Can you work these out from the model? Positions are in its coordinate system, mm. Give positions to 0.01 mm unless a question says otherwise; leave off trailing zeros. Order: outer loops, then holes, each group sorted by start corner. A loop starts at its lowest first (then second) coordinate and runs counter-clockwise, first axis right, second up. Notation, with made-up numbers: M -1.5,-29.75 L 3.5,-29.75 A21 ccw 3.5,-19.75 Z; hole C 72,-34 d9. An arc over 180 degrees is marked long. One line per question, with ' | ' between items. Start each with the question number.
1) If we section it at A-A, the plane y = 6: Please give me the cut outline in (x, z), plus the area to 3 significant figures.
2) Please list where these lines run through material, in increasing order: line 1 along Z through (x, y) = (28, 2.75); line 2 along X through (y, z) = (7, -58); line 3 along Y through (x, z) = (18.5, -72). Write a range as [from, to].
3) I'm going to push flat-ended pins straight in: pin 1 Ø12 at (x, z) = (62.5, -54.5) entering from -Y; pin 2 Ø2 at (y, z) = (1, -73.5) entering from +X; pin 3 Ø4 at (x, y) = (25, 3.5) entering from +Z; pin 4 Ø5 at (y, z) = (8, -38) entering from -X. Where does each tip first touch, or does it pass through?
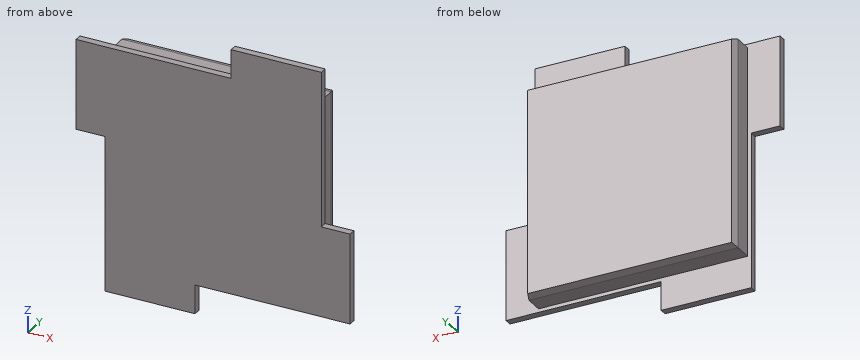
```python
from build123d import *

# Parameters (mm, degrees)
ESQUISSE1_W        = 8
ESQUISSE1_H        = 25
ESQUISSE1_W_2      = 25
ESQUISSE1_H_2      = 8
ESQUISSE1_W_3      = 60
ESQUISSE1_H_3      = 60
BOSS_EXTRU_1_DEPTH = 2
ESQUISSE2_W        = 58
ESQUISSE2_H        = 58
BOSS_EXTRU_2_DEPTH = 5
BOSS_EXTRU_3_START = 5
ESQUISSE2_3_W      = 58
ESQUISSE2_3_H      = 58
BOSS_EXTRU_3_DEPTH = 2
BOSS_EXTRU_3_TAPER = 20


with BuildPart() as part:
    # Esquisse1 → Boss.-Extru.1 (new body)
    with BuildSketch(Plane(origin=(0, 0, 0), x_dir=(1, 0, 0), z_dir=(0, 1, 0))):
        with Locations((4, 20.5)):
            Rectangle(ESQUISSE1_W, ESQUISSE1_H)
        with Locations((20.5, 72)):
            Rectangle(ESQUISSE1_W_2, ESQUISSE1_H_2)
        with Locations((72, 55.5)):
            Rectangle(ESQUISSE1_W, ESQUISSE1_H)
        with Locations((55.5, 4)):
            Rectangle(ESQUISSE1_W_2, ESQUISSE1_H_2)
        with Locations((38, 38)):
            Rectangle(ESQUISSE1_W_3, ESQUISSE1_H_3)
    extrude(amount=BOSS_EXTRU_1_DEPTH)

    # Esquisse2 → Boss.-Extru.2 (add)
    with BuildSketch(Plane(origin=(0, 2, 0), x_dir=(1, 0, 0), z_dir=(0, 1, 0))):
        with Locations((38, 38)):
            Rectangle(ESQUISSE2_W, ESQUISSE2_H)
    extrude(amount=BOSS_EXTRU_2_DEPTH)

    # Esquisse2_3 → Boss.-Extru.3 (add)
    with BuildSketch(Plane(origin=(0, 2, 0), x_dir=(1, 0, 0), z_dir=(0, 1, 0)).offset(BOSS_EXTRU_3_START)):
        with Locations((38, 38)):
            Rectangle(ESQUISSE2_3_W, ESQUISSE2_3_H)
    extrude(amount=BOSS_EXTRU_3_DEPTH, taper=BOSS_EXTRU_3_TAPER)


solid = part.part
```
Results found:
1) outline: M 9,-67 L 67,-67 L 67,-9 L 9,-9 Z | area: 3,360 mm²
2) line 1: z = [-67, -9] | line 2: x = [9, 67] | line 3: y = [0, 2]
3) pin 1: stops at y = 0 | pin 2: stops at x = 33 | pin 3: stops at z = -8 | pin 4: stops at x = 9
